from build123d import *

# Parameters (mm, degrees)
SKETCH_1_W          = 66
SKETCH_1_H          = 43
SKETCH_1_W_2        = 60
SKETCH_1_H_2        = 37
EXTRUDE_1_DEPTH     = 26
SKETCH_2_W          = 66
SKETCH_2_H          = 43
EXTRUDE_2_DEPTH     = 3
EXTRUDE_3_DEPTH     = 40
CUT_EXTRUDE_1_REACH = 45
SKETCH_4_W          = 10
SKETCH_4_H          = 3
SKETCH_6_R          = 2.5
SKETCH_6_R_2        = 1.45
EXTRUDE_5_DEPTH     = 5
CUT_EXTRUDE_2_REACH = 31
FILLET_1_R          = 3
FILLET_2_R          = 3


with BuildPart() as part:
    # 草图1 → 凸台-拉伸1 (new body)
    with BuildSketch(Plane.XY):
        with Locations((-0.837138389, -4.179180765)):
            Rectangle(SKETCH_1_W, SKETCH_1_H)
        with Locations((-0.837138389, -4.179180765)):
            Rectangle(SKETCH_1_W_2, SKETCH_1_H_2, mode=Mode.SUBTRACT)
    extrude(amount=EXTRUDE_1_DEPTH)

    # 草图2 → 凸台-拉伸2 (add)
    with BuildSketch(Plane(origin=(0, 0, 0), x_dir=(-1, 0, 0), z_dir=(0, 0, -1))):
        with Locations((0.837138389, -4.179180765)):
            Rectangle(SKETCH_2_W, SKETCH_2_H)
    extrude(amount=EXTRUDE_2_DEPTH)

    # 草图3 → 凸台-拉伸3 (add)
    with BuildSketch(Plane(origin=(0, 17.320819235, 0), x_dir=(1, 0, 0), z_dir=(0, 1, 0))):
        Polygon((-21.837138389, -26), (-21.837138389, -23), (-11.837138389, -23), (-11.837138389, -26), (22.162861611, -26), (22.162861611, -22), (-23.837138389, -22), (-23.837138389, -26), align=None)
    extrude(amount=EXTRUDE_3_DEPTH)

    # 草图4 → 切除-拉伸1 (cut, up to next)
    with BuildSketch(Plane(origin=(0, 17.320819235, 0), x_dir=(1, 0, 0), z_dir=(0, 1, 0)), mode=Mode.PRIVATE) as cut_extrude_1_sk1:
        with Locations((-16.837138389, -24.5)):
            Rectangle(SKETCH_4_W, SKETCH_4_H)
    cut_extrude_1_tool1 = extrude(cut_extrude_1_sk1.sketch, amount=-CUT_EXTRUDE_1_REACH, mode=Mode.PRIVATE) & part.part
    add(cut_extrude_1_tool1.solids().sort_by_distance((-16.837138, 17.320819, 24.5))[0], mode=Mode.SUBTRACT)

    # 草图6 → 凸台-拉伸5 (add)
    with BuildSketch(Plane.XY):
        with Locations((24.812861611, -18.829180765)):
            Circle(SKETCH_6_R)
        with Locations((24.812861611, -18.829180765)):
            Circle(SKETCH_6_R_2, mode=Mode.SUBTRACT)
        with Locations((-26.487138389, -18.829180765)):
            Circle(SKETCH_6_R)
        with Locations((-26.487138389, -18.829180765)):
            Circle(SKETCH_6_R_2, mode=Mode.SUBTRACT)
        with Locations((24.812861611, 10.470819235)):
            Circle(SKETCH_6_R)
        with Locations((24.812861611, 10.470819235)):
            Circle(SKETCH_6_R_2, mode=Mode.SUBTRACT)
        with Locations((-26.487138389, 10.470819235)):
            Circle(SKETCH_6_R)
        with Locations((-26.487138389, 10.470819235)):
            Circle(SKETCH_6_R_2, mode=Mode.SUBTRACT)
    extrude(amount=EXTRUDE_5_DEPTH)

    # 草图10 → 切除-拉伸2 (cut, up to next)
    with BuildSketch(Plane.XY.offset(26), mode=Mode.PRIVATE) as cut_extrude_2_sk1:
        with BuildLine():
            Line((2.162861611, 26.320819235), (22.162861611, 26.320819235))
            Line((22.162861611, 26.320819235), (22.162861611, 48.320819235))
            Line((22.162861611, 48.320819235), (2.162861611, 48.320819235))
            ThreePointArc((2.162861611, 48.320819235), (-8.837138389, 37.320819235), (2.162861611, 26.320819235))
        make_face()
    cut_extrude_2_tool1 = extrude(cut_extrude_2_sk1.sketch, amount=-CUT_EXTRUDE_2_REACH, mode=Mode.PRIVATE) & part.part
    add(cut_extrude_2_tool1.solids().sort_by_distance((7.737936, 37.320819, 26))[0], mode=Mode.SUBTRACT)

    # 圆角1
    fillet_1_edges = [part.edges().sort_by_distance(p)[0] for p in [
        (32.162861611, -4.179180765, -3),
        (-0.837138389, -25.679180765, -3),
        (-33.837138389, -4.179180765, -3),
        (-0.837138389, 17.320819235, -3),
        (32.162861611, -25.679180765, 11.5),
        (-33.837138389, -25.679180765, 11.5),
        (-33.837138389, 17.320819235, 11.5),
        (32.162861611, 17.320819235, 11.5),
    ]]
    fillet(fillet_1_edges, radius=FILLET_1_R)

    # 圆角2
    fillet_2_edges = [part.edges().sort_by_distance(p)[0] for p in [
        (-23.837138389, 17.320819235, 24),
        (22.162861611, 17.320819235, 24),
        (-0.837138389, 17.320819235, 22),
    ]]
    fillet(fillet_2_edges, radius=FILLET_2_R)


solid = part.part
Build history of the part. All positions in model axes, mm. A direction names the side the tool comes from. Coordinates: 2 decimals unless noted, no trailing zeros. Order: outer loops, then holes, each group sorted by start corner. A loop starts at its lowest first (then second) coordinate and runs counter-clockwise, first axis right, second up. Notation, with made-up numbers: (62, 45.5) - (98, 45.5) arc R10 ccw to (98, 49.5) - close; hole circle Ø6 at (73, 34). An arc over 180 degrees is marked (long way). Write item = value, one per line. Start each with the question number.
1) Saw through at A-A on z = 13.5. Write the cut outline in (x, y), then the cut area to 3 significant figures.
2) Wall check: line 1 along Y through (x, z) = (16, 15.75); line 2 along X through (y, z) = (11, 18); line 3 along Y through (x, z) = (-2, 23). Give the ranges that are in metal, low to high. Write a range as from..to.
3) Saw through at C-C on y = 1. Write the cut outline in (x, z), then the cut area to 3 significant figures.
4) Flat gauge pins, fed straight in: pin 1 Ø2 at (y, z) = (24, 25) entering from +X; pin 2 Ø5 at (x, y) = (25, 18) entering from +Z; pin 3 Ø8 at (x, z) = (11.5, 1) entering from +Y; pin 4 Ø10 at (x, y) = (-14, 23) entering from -Z. Where does each tip first touch, or does it go through?
5) Saw through at D-D on y = 18.5. Write the cut outline in (x, z).
6) Saw through at B-B on x = 5. Write the cut outline in (y, z), then the cut area to 3 significant figures.
7) Two-plate mould, pull along Y, no slides. Class faces 1 (the face through (25, 10, 0)), 2 (the face through (26, -20, 5)), 3 (the face through (0, -25.679, 13)), 4 (the face through (22.163, 23, 24)): pulls with the +Y half, pulls with the -Y half, needs draft (parallel to the pull), parting line crosses it, or undercut.
8) 3-axis set-ups, long thin cutter, end or side, ignore diameter. For faces 5 (the face through (23.744, 11.451, 2.465)), 6 (the face through (-32.94, -24.82, 12.82)), 7 (the face through (0, -4, -3)), 8 (the face through (22.163, 53, 24)), 9 (the face through (-11, 39, 22)): which of +Z, -Z, +X, -X, +Y, -Y reach the whole face in a straight line?
From the geometry:
q1.outline = (-33.84, -22.68) arc R3 ccw to (-30.84, -25.68) - (29.16, -25.68) arc R3 ccw to (32.16, -22.68) - (32.16, 14.32) arc R3 ccw to (29.16, 17.32) - (-30.84, 17.32) arc R3 ccw to (-33.84, 14.32) - close; hole (-30.84, -22.68) - (29.16, -22.68) - (29.16, 14.32) - (-30.84, 14.32) - close
q1.area = 610 mm^2
q2.line_1 = -25.68..-22.68, 14.32..17.32
q2.line_2 = -33.84..-30.84, 29.16..32.16
q2.line_3 = -25.68..-22.68, 14.32..27.14, 47.5..57.32
q3.outline = (-33.84, 0) arc R3 ccw to (-30.84, -3) - (29.16, -3) arc R3 ccw to (32.16, 0) - (32.16, 26) - (29.16, 26) - (29.16, 0) - (-30.84, 0) - (-30.84, 26) - (-33.84, 26) - close
q3.area = 350 mm^2
q4.pin_1 = 22.16
q4.pin_2 = 26
q4.pin_3 = 17.32
q4.pin_4 = 20.9
q5.outline = (-24.45, 21.38) - (22.78, 21.38) - (22.78, 26) - (-11.84, 26) - (-11.84, 23) - (-21.84, 23) - (-21.84, 26) - (-24.45, 26) - close
q6.outline = (-25.68, 0) arc R3 ccw to (-22.68, -3) - (14.32, -3) arc R3 ccw to (17.32, 0) - (17.32, 19) arc R3 cw to (20.32, 22) - (26.32, 22) - (26.32, 26) - (14.32, 26) - (14.32, 0) - (-22.68, 0) - (-22.68, 26) - (-25.68, 26) - close; (48.32, 22) - (57.32, 22) - (57.32, 26) - (48.32, 26) - close
q6.area = 355 mm^2
q7.face_1 = undercut
q7.face_2 = undercut
q7.face_3 = pulls with the -Y half
q7.face_4 = needs draft
q8.face_5 = +Z
q8.face_6 = +Z, -Z, -X, -Y
q8.face_7 = -Z, +X, -X, +Y, -Y
q8.face_8 = +Z, -Z, +X, +Y
q8.face_9 = -Z, +X, -X, +Y
